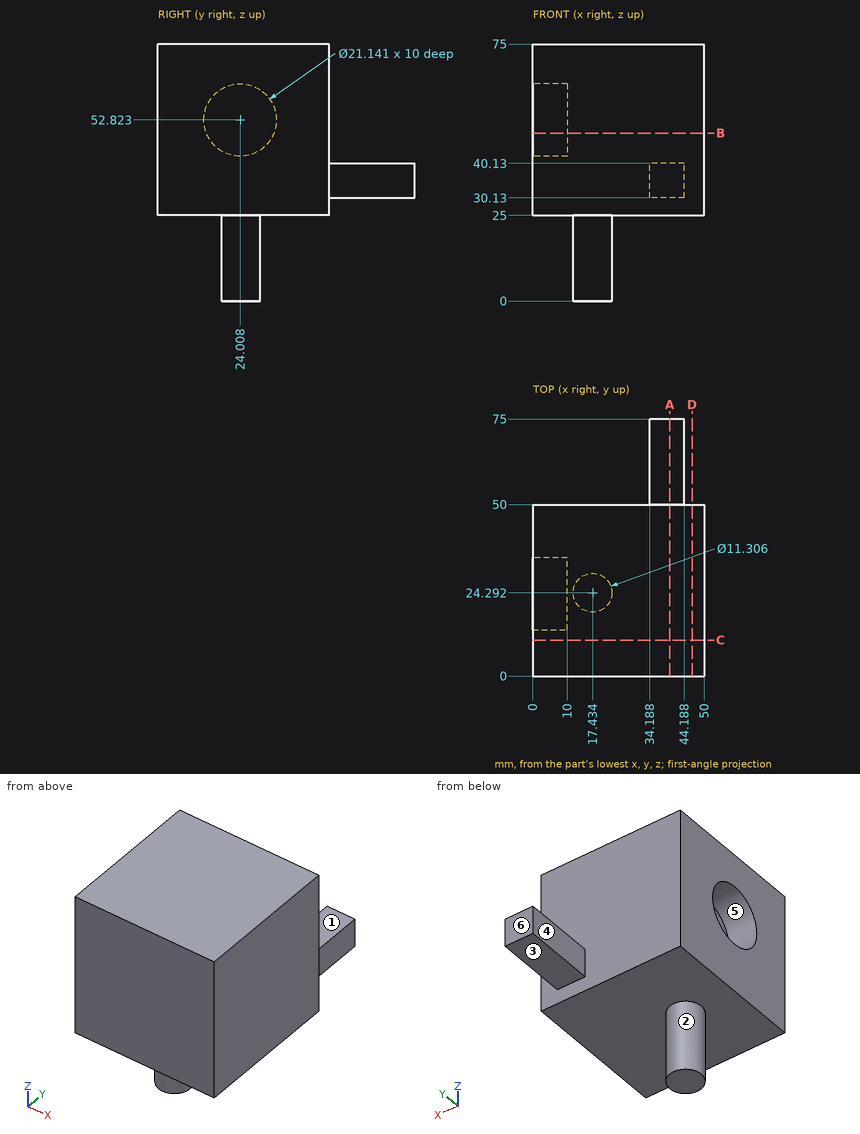
Could you check a few things on this drawing? It's one solid part, dimensions in mm from its lowest x, y, z. A direction names the side the tool comes from. Coordinates: 2 decimals unless noted, no trailing zeros. Write each loop counter-clockwise with the first axis right and the second up, starting at its lowest first coordinate (ties: lowest second). Pieces come first, ordered by that corner, then holes. Notation, with made-up numbers: (-21.75, 21.5) - (22.25, 21.5) arc R20 cw to (22.25, 45.5) - close; hole circle Ø6 at (86, -11.5). An arc over 180 degrees is marked (long way). Return JSON: item names as keys, results as strings. Group by question number.
Item 1: Please list where these lines run through material, in increasing order: probe 1 along Z at (x, y) = (40, 7.5); probe 2 along Z at (x, y) = (3, 24); probe 3 along Y at (x, z) = (41, 55).
Item 2: If we section it at C-C (y = 10.5): Write out the boundary of the cut face in (x, z).
Item 3: If we section it at A-A (x = 40): Write out the boundary of the cut face in (y, z), then the cut area to 3 significant figures.
Item 4: I'm going to push flat-ended pins straight in: pin 1 Ø8 at (x, y) = (40.5, 68.5) entering from -Z; pin 2 Ø10.5 at (y, z) = (26, 48) entering from -X; pin 3 Ø15 at (x, y) = (32.5, 33) entering from -Z. Where does each tip first touch, or does it pass through?
Item 5: If we section it at B-B (z = 49): Write out the boundary of the cut face in (x, y).
Item 6: Which directions (+Z, -Z, +X, -X, +Y, -Y) give clear straight access to the entire face, cutting with the end or side of a thin tool? Please do the marked faces 1, 2 and 3.
Item 7: We'd pull the mould along Y, two halves only. Please class the marked faces 4, 5 and 6: pulls with the +Y half, pulls with the -Y half, needs draft (parallel to the pull), parting line crosses it, or undercut.
Return value:
{
 "1": {"probe 1": "z = 25 to 75", "probe 2": "z = 25 to 42.25, 63.39 to 75", "probe 3": "y = 0 to 50"},
 "2": {"outline": "(0, 25) - (50, 25) - (50, 75) - (0, 75) - close"},
 "3": {"outline": "(0, 25) - (50, 25) - (50, 30.13) - (75, 30.13) - (75, 40.13) - (50, 40.13) - (50, 75) - (0, 75) - close", "area": "2,750 mm^2"},
 "4": {"pin 1": "stops at z = 30.13", "pin 2": "stops at x = 10", "pin 3": "stops at z = 25"},
 "5": {"outline": "(0, 0) - (50, 0) - (50, 50) - (0, 50) - (0, 33.86) - (10, 33.86) - (10, 14.15) - (0, 14.15) - close"},
 "6": {"face 1": "+Z, +X, -X, +Y", "face 2": "-Z", "face 3": "-Z, +X, -X, +Y"},
 "7": {"face 4": "needs draft", "face 5": "undercut", "face 6": "pulls with the +Y half"}
}
